Part model, mm, in its own coordinate system. A direction names the side the tool comes from. Round coordinates to 2 decimals unless told otherwise and drop trailing zeros. Loops run counter-clockwise (first coordinate to the right, second up) from the corner with the lowest first, then second, coordinate; pieces in that order, holes last.
(1) Flat gauge pins, fed straight in: pin 1 (12.5 mm diameter, centred on x = 18.5, z = 16.5, fed in from -Y); pin 2 (1.6 mm diameter, centred on x = 23, y = 8, fed in from +Z); pin 3 (20.5 mm diameter, centred on x = 22, y = 56.5, fed in from +Z); pin 4 (7.5 mm diameter, centred on x = 16, y = 45, fed in from +Z). Where does each tip first touch, or does it go through?
(2) Cut at C-C on y = 30.5. List the corners of the cut face in (x, z).
(3) Cut at A-A on z = 22.5. List the corners of the cut face in (x, y).
(4) Tool access for faces 1 (the face through (16, 8, 3)), 2 (the face through (0, 71, 14)), 3 (the face through (25.7, 9, 5)): list every direction of +Z, -Z, +X, -X, +Y, -Y with a clear straight run to the whole face (end or side of a thin tool).
(5) Mould opens along Z. For faces 4 (the face through (18.7, 9, 5)), 5 (the face through (19, 71, 0)), 6 (the face through (23, 8, 3)), 7 (the face through (33, 70, 28.4)) say: +Z half, -Z half, draft (parallel to the pull), parting line (faces both ways), or undercut.
(6) Cut at B-B on z = 9.25. List the corners of the cut face in (x, y), then the cut area to 3 significant figures.
(7) Probe probe 1 along X at (y, z) = (81.5, 17.5); probe 2 along X at (y, z) = (59, 11.75); probe 3 along Y at (x, z) = (23, 12.5). List the from-to ranges inside material, lowest first.
Autodesk Fusion 360 part; units mm, degrees
sketch "Sketch1" plane through (0, 0, 0) normal (0, 0, 1) x (1, 0, 0)
  line L0 (0, 0) -> (39.4, 0)
  line L1 (39.4, 0) -> (39.4, 141)
  line L2 (39.4, 141) -> (0, 141)
  line L3 (0, 141) -> (0, 0)
  line L4 (7, 7) -> (32.4, 7)
  line L5 (32.4, 7) -> (32.4, 134)
  line L6 (32.4, 134) -> (7, 134)
  line L7 (7, 134) -> (7, 7)
  line L8 (10, 10) -> (29.4, 10)
  line L9 (29.4, 10) -> (29.4, 131)
  line L10 (29.4, 131) -> (10, 131)
  line L11 (10, 131) -> (10, 10)
  line L12 (11, 11) -> (28.4, 11)
  line L13 (28.4, 11) -> (28.4, 130)
  line L14 (28.4, 130) -> (11, 130)
  line L15 (11, 130) -> (11, 11)
  dimension "d1" = 39.4
  dimension "d2" = 141
  dimension "d3" = 25.4
  dimension "d4" = 127
  dimension "d5" = 7
  dimension "d6" = 7
  dimension "d7" = 19.4
  dimension "d8" = 121
  dimension "d9" = 3
  dimension "d10" = 3
  dimension "d11" = 17.4
  dimension "d12" = 119
  dimension "d13" = 1
  dimension "d14" = 1
extrude "Extrude1" add sketch "Sketch1" along normal blind 1 contours L0 L1 L2 L3 | L4 L5 L6 L7 | L8 L9 L10 L11 | L12 L13 L14 L15
sketch "Sketch2" plane through (0, 0, 1) normal (0, 0, 1) x (-1, 0, 0)
  line L0 (0, -141) -> (0, 0)
  line L1 (0, 0) -> (-39.4, 0)
  line L2 (-39.4, 0) -> (-39.4, -141)
  line L3 (-39.4, -141) -> (0, -141)
  line L4 (-7, -7) -> (-32.4, -7)
  line L5 (-32.4, -7) -> (-32.4, -134)
  line L6 (-32.4, -134) -> (-7, -134)
  line L7 (-7, -134) -> (-7, -7)
  line L8 (-10, -10) -> (-29.4, -10)
  line L9 (-29.4, -10) -> (-29.4, -131)
  line L10 (-29.4, -131) -> (-10, -131)
  line L11 (-10, -131) -> (-10, -10)
  line L12 (-11, -11) -> (-28.4, -11)
  line L13 (-28.4, -11) -> (-28.4, -130)
  line L14 (-28.4, -130) -> (-11, -130)
  line L15 (-11, -130) -> (-11, -11)
  dimension "d17" = 25.4
  dimension "d18" = 127
  dimension "d19" = 19.4
  dimension "d20" = 121
  dimension "d21" = 17.4
  dimension "d22" = 119
  dimension "d23" = 7
  dimension "d24" = 7
  dimension "d25" = 3
  dimension "d26" = 3
  dimension "d27" = 1
  dimension "d28" = 1
extrude "Extrude2" add sketch "Sketch2" along normal blind 12 draft -1 contours L12 L13 L14 L15
sketch "Sketch3" plane through (0, 0, 1) normal (0, 0, 1) x (-1, 0, 0)
  line L0 (-11, -130) -> (-28.4, -130)
  line L1 (-28.4, -130) -> (-28.4, -11)
  line L2 (-28.4, -11) -> (-11, -11)
  line L3 (-11, -11) -> (-11, -130)
  line L4 (0, -141) -> (0, 0)
  line L5 (0, 0) -> (-39.4, 0)
  line L6 (-39.4, 0) -> (-39.4, -141)
  line L7 (-39.4, -141) -> (0, -141)
  line L8 (-7, -7) -> (-32.4, -7)
  line L9 (-32.4, -7) -> (-32.4, -134)
  line L10 (-32.4, -134) -> (-7, -134)
  line L11 (-7, -134) -> (-7, -7)
  dimension "d31" = 25.4
  dimension "d32" = 127
  dimension "d33" = 7
  dimension "d34" = 7
extrude "Extrude3" add sketch "Sketch3" along normal blind 25.4 contours L4 L5 L6 L7
sketch "Sketch4" plane through (0, 0, 1) normal (0, 0, 1) x (-1, 0, 0)
  line L0 (-7, -7) -> (-32.4, -7)
  line L1 (-32.4, -7) -> (-32.4, -134)
  line L2 (-32.4, -134) -> (-7, -134)
  line L3 (-7, -134) -> (-7, -7)
  line L4 (-11, -130) -> (-28.4, -130)
  line L5 (-28.4, -130) -> (-28.4, -11)
  line L6 (-28.4, -11) -> (-11, -11)
  line L7 (-11, -11) -> (-11, -130)
  line L8 (-10, -10) -> (-29.4, -10)
  line L9 (-29.4, -10) -> (-29.4, -131)
  line L10 (-29.4, -131) -> (-10, -131)
  line L11 (-10, -131) -> (-10, -10)
  dimension "d37" = 19.4
  dimension "d38" = 121
  dimension "d39" = 3
  dimension "d40" = 3
extrude "Extrude4" add sketch "Sketch4" along normal blind 24.4 draft -1 contours L8 L9 L10 L11
extrude "Extrude5" add 1 faces at (2.3333, 49.3333, 26.4) along direction (0, 0, 1) blind 2
sketch "Sketch5" plane through (0, 9.9795, -0.1742) normal (0, -0.9998, 0.0175) x (1, 0, 0)
  line L0 (28.9741, 25.5781) -> (10.4259, 25.5781)
  line L1 (10.4259, 25.5781) -> (10, 1.1744)
  line L2 (10, 1.1744) -> (29.4, 1.1744)
  line L3 (29.4, 1.1744) -> (28.9741, 25.5781)
sketch "Sketch6" plane through (0, 7, 0) normal (0, 1, 0) x (-1, 0, 0)
  line L0 (-32.4, 1) -> (-7, 1)
  line L1 (-7, 1) -> (-7, 28.4)
  line L2 (-7, 28.4) -> (-32.4, 28.4)
  line L3 (-32.4, 28.4) -> (-32.4, 1)
  line L4 (-25.7, 8) -> (-20.7, 8)
  line L5 (-20.7, 8) -> (-20.7, 3)
  line L6 (-20.7, 3) -> (-25.7, 3)
  line L7 (-25.7, 3) -> (-25.7, 8)
  line L8 (-19.7, 28.4) -> (-19.7, -1.222)
  line L9 (-10, 1) -> (-29.4, 1)
  dimension "d45" = 5
  dimension "d46" = 5
  dimension "d47" = 1
  dimension "d48" = 2
extrude "Extrude6" add sketch "Sketch6" along normal blind 3.5 contours L4 L5 L6 L7
sketch "Sketch7" plane through (0, 7, 0) normal (0, 1, 0) x (-1, 0, 0)
  line L0 (-25.7, 3) -> (-25.7, 8)
  line L1 (-25.7, 8) -> (-20.7, 8)
  line L2 (-20.7, 8) -> (-20.7, 3)
  line L3 (-20.7, 3) -> (-25.7, 3)
  line L4 (-32.4, 1) -> (-7, 1)
  line L5 (-7, 1) -> (-7, 28.4)
  line L6 (-7, 28.4) -> (-32.4, 28.4)
  line L7 (-32.4, 28.4) -> (-32.4, 1)
  line L8 (-19.7, 28.4) -> (-19.7, 1)
  line L9 (-18.7, 8) -> (-13.7, 8)
  line L10 (-13.7, 8) -> (-13.7, 3)
  line L11 (-13.7, 3) -> (-18.7, 3)
  line L12 (-18.7, 3) -> (-18.7, 8)
  line L13 (-10, 1) -> (-29.4, 1)
  dimension "d51" = 5
  dimension "d52" = 5
  dimension "d53" = 1
  dimension "d54" = 2
extrude "Extrude7" add sketch "Sketch7" along normal blind 3.5 contours L9 L10 L11 L12
Final values:
1. pin 1: stops at y = 0
1. pin 2: stops at z = 8
1. pin 3: stops at z = 25.4
1. pin 4: stops at z = 13
2. outline: (0, 0) - (39.4, 0) - (39.4, 28.4) - (32.4, 28.4) - (32.4, 1) - (29.4, 1) - (28.97, 25.4) - (28.83, 25.4) - (28.4, 1) - (28.19, 13) - (11.21, 13) - (11, 1) - (10.57, 25.4) - (10.43, 25.4) - (10, 1) - (7, 1) - (7, 28.4) - (0, 28.4) - close
3. outline: (0, 0) - (39.4, 0) - (39.4, 141) - (0, 141) - close; (10.38, 10.38) - (29.02, 10.38) - (29.02, 130.62) - (10.38, 130.62) - close; hole (7, 7) - (32.4, 7) - (32.4, 134) - (7, 134) - close; hole (10.62, 10.62) - (28.78, 10.62) - (28.78, 130.38) - (10.62, 130.38) - close
4. face 1: none
4. face 2: +Z, -Z, -X, +Y, -Y
4. face 3: +Z
5. face 4: draft
5. face 5: -Z half
5. face 6: undercut
5. face 7: +Z half
6. outline: (0, 0) - (39.4, 0) - (39.4, 141) - (0, 141) - close; (10.14, 10.14) - (29.26, 10.14) - (29.26, 130.86) - (10.14, 130.86) - close; (11.14, 11.14) - (28.26, 11.14) - (28.26, 129.86) - (11.14, 129.86) - close; hole (7, 7) - (32.4, 7) - (32.4, 134) - (7, 134) - close; hole (10.86, 10.86) - (28.54, 10.86) - (28.54, 130.14) - (10.86, 130.14) - close
6. area: 4,560 mm2
7. probe 1: x = 0 to 7, 10.29 to 10.71, 28.69 to 29.11, 32.4 to 39.4
7. probe 2: x = 0 to 7, 10.19 to 10.81, 11.19 to 28.21, 28.59 to 29.21, 32.4 to 39.4
7. probe 3: y = 0 to 7, 10.2 to 10.8, 11.2 to 129.8, 130.2 to 130.8, 134 to 141
